from build123d import *

# Parameters (mm, degrees)
F0_R     = 15.875
F1_DEPTH = 12.7


with BuildPart() as f1:
    # F0 (on Top) → F1 (new body)
    with BuildSketch(Plane.XY):
        with BuildLine():
            ThreePointArc((139.501369, -7.447021), (139.650333, -3.724835), (139.7, 0))
            ThreePointArc((139.7, 0), (139.650333, 3.724835), (139.501369, 7.447021))
            ThreePointArc((139.501369, 7.447021), (132.862595, 43.169674), (117.236227, 75.97208))
            ThreePointArc((117.236227, 75.97208), (113.019674, 82.1136), (108.481729, 88.021614))
            ThreePointArc((108.481729, 88.021614), (82.1136, 113.019674), (50.190832, 130.37243))
            ThreePointArc((50.190832, 130.37243), (43.169674, 132.862595), (36.025756, 134.974942))
            ThreePointArc((36.025756, 134.974942), (0, 139.7), (-36.025756, 134.974942))
            ThreePointArc((-36.025756, 134.974942), (-43.169674, 132.862595), (-50.190832, 130.37243))
            ThreePointArc((-50.190832, 130.37243), (-82.1136, 113.019674), (-108.481729, 88.021614))
            ThreePointArc((-108.481729, 88.021614), (-113.019674, 82.1136), (-117.236227, 75.97208))
            ThreePointArc((-117.236227, 75.97208), (-132.862595, 43.169674), (-139.501369, 7.447021))
            ThreePointArc((-139.501369, 7.447021), (-139.7, 0), (-139.501369, -7.447021))
            ThreePointArc((-139.501369, -7.447021), (-132.862595, -43.169674), (-117.236227, -75.97208))
            ThreePointArc((-117.236227, -75.97208), (-113.019674, -82.1136), (-108.481729, -88.021614))
            ThreePointArc((-108.481729, -88.021614), (-82.1136, -113.019674), (-50.190832, -130.37243))
            ThreePointArc((-50.190832, -130.37243), (-43.169674, -132.862595), (-36.025756, -134.974942))
            ThreePointArc((-36.025756, -134.974942), (0, -139.7), (36.025756, -134.974942))
            ThreePointArc((36.025756, -134.974942), (43.169674, -132.862595), (50.190832, -130.37243))
            ThreePointArc((50.190832, -130.37243), (82.1136, -113.019674), (108.481729, -88.021614))
            ThreePointArc((108.481729, -88.021614), (113.019674, -82.1136), (117.236227, -75.97208))
            ThreePointArc((117.236227, -75.97208), (132.862595, -43.169674), (139.501369, -7.447021))
        make_face()
        Circle(F0_R, mode=Mode.SUBTRACT)
        with BuildLine():
            ThreePointArc((117.236227, 75.97208), (132.862595, 43.169674), (139.501369, 7.447021))
            Line((139.501369, 7.447021), (160.943947, 38.940288))
            Line((160.943947, 38.940288), (157.019431, 51.018706))
            Line((157.019431, 51.018706), (153.094915, 63.097124))
            Line((153.094915, 63.097124), (117.236227, 75.97208))
        make_face()
        with BuildLine():
            Line((160.943947, -38.940288), (139.501369, -7.447021))
            ThreePointArc((139.501369, -7.447021), (132.862595, -43.169674), (117.236227, -75.97208))
            Line((117.236227, -75.97208), (153.094915, -63.097124))
            Line((153.094915, -63.097124), (157.019431, -51.018706))
            Line((157.019431, -51.018706), (160.943947, -38.940288))
        make_face()
        with BuildLine():
            ThreePointArc((50.190832, 130.37243), (82.1136, 113.019674), (108.481729, 88.021614))
            Line((108.481729, 88.021614), (107.317861, 126.103833))
            Line((107.317861, 126.103833), (97.043345, 133.568706))
            Line((97.043345, 133.568706), (86.768829, 141.033578))
            Line((86.768829, 141.033578), (50.190832, 130.37243))
        make_face()
        with BuildLine():
            Line((107.317861, -126.103833), (108.481729, -88.021614))
            ThreePointArc((108.481729, -88.021614), (82.1136, -113.019674), (50.190832, -130.37243))
            Line((50.190832, -130.37243), (86.768829, -141.033578))
            Line((86.768829, -141.033578), (97.043345, -133.568706))
            Line((97.043345, -133.568706), (107.317861, -126.103833))
        make_face()
        with BuildLine():
            ThreePointArc((-36.025756, 134.974942), (0, 139.7), (36.025756, 134.974942))
            Line((36.025756, 134.974942), (12.7, 165.1))
            Line((12.7, 165.1), (0, 165.1))
            Line((0, 165.1), (-12.7, 165.1))
            Line((-12.7, 165.1), (-36.025756, 134.974942))
        make_face()
        with BuildLine():
            Line((12.7, -165.1), (36.025756, -134.974942))
            ThreePointArc((36.025756, -134.974942), (0, -139.7), (-36.025756, -134.974942))
            Line((-36.025756, -134.974942), (-12.7, -165.1))
            Line((-12.7, -165.1), (0, -165.1))
            Line((0, -165.1), (12.7, -165.1))
        make_face()
        with BuildLine():
            ThreePointArc((-108.481729, 88.021614), (-82.1136, 113.019674), (-50.190832, 130.37243))
            Line((-50.190832, 130.37243), (-86.768829, 141.033578))
            Line((-86.768829, 141.033578), (-97.043345, 133.568706))
            Line((-97.043345, 133.568706), (-107.317861, 126.103833))
            Line((-107.317861, 126.103833), (-108.481729, 88.021614))
        make_face()
        with BuildLine():
            Line((-86.768829, -141.033578), (-50.190832, -130.37243))
            ThreePointArc((-50.190832, -130.37243), (-82.1136, -113.019674), (-108.481729, -88.021614))
            Line((-108.481729, -88.021614), (-107.317861, -126.103833))
            Line((-107.317861, -126.103833), (-97.043345, -133.568706))
            Line((-97.043345, -133.568706), (-86.768829, -141.033578))
        make_face()
        with BuildLine():
            ThreePointArc((-139.501369, 7.447021), (-132.862595, 43.169674), (-117.236227, 75.97208))
            Line((-117.236227, 75.97208), (-153.094915, 63.097124))
            Line((-153.094915, 63.097124), (-157.019431, 51.018706))
            Line((-157.019431, 51.018706), (-160.943947, 38.940288))
            Line((-160.943947, 38.940288), (-139.501369, 7.447021))
        make_face()
        with BuildLine():
            Line((-153.094915, -63.097124), (-117.236227, -75.97208))
            ThreePointArc((-117.236227, -75.97208), (-132.862595, -43.169674), (-139.501369, -7.447021))
            Line((-139.501369, -7.447021), (-160.943947, -38.940288))
            Line((-160.943947, -38.940288), (-157.019431, -51.018706))
            Line((-157.019431, -51.018706), (-153.094915, -63.097124))
        make_face()
    extrude(amount=F1_DEPTH)


solid = f1.part
Can you work these out from the model? Positions are in its coordinate system, mm. A direction names the side the tool comes from. Give positions to 0.01 mm unless a question says otherwise; leave off trailing zeros. Loops run counter-clockwise (first coordinate to the right, second up) from the corner with the lowest first, then second, coordinate; pieces in that order, holes last. Notation, with made-up numbers: (60.25, 48) - (108.25, 48) arc R33 cw to (108.25, 77) - close; hole circle Ø1 at (16, 8). An arc over 180 degrees is marked (long way). Return JSON: item names as keys, results as strings.
1. We'd pull the mould along Y, two halves only. Please class faces 1 (the face through (-139.7, 0.1, 6.3)), 2 (the face through (-134.915, 69.625, 6.261)), 3 (the face through (156.964, -51.188, 6.261)): +Y half, -Y half, draft (parallel to the pull), parting line (faces both ways), or undercut.
Output values:
{"face 1": "undercut", "face 2": "+Y half", "face 3": "-Y half"}
2. For faces 4 (the face through (-43.27, -132.83, 6.26)), 5 (the face through (24.526, 149.827, 6.261)), 6 (the face through (-150.07, -22.97, 6.26)), 7 (the face through (150.07, 22.97, 6.26)), which set-ups out of +Z, -Z, +X, -X, +Y, -Y let a thin tool reach every point of the face, with its end or its side?
Output values:
{"face 4": "+Z, -Z, -Y", "face 5": "+Z, -Z, +Y", "face 6": "+Z, -Z, -X", "face 7": "+Z, -Z, +X"}
3. I'm going to push flat-ended pins straight in: pin 1 Ø6 at (x, z) = (20.5, 11.5) entering from +Y; pin 2 Ø3 at (y, z) = (-35, 7) entering from +X; pin 3 Ø4 at (y, z) = (-57, 10) entering from +X. Where does each tip first touch, or does it pass through?
Output values:
{"pin 1": "stops at y = 158.9", "pin 2": "stops at x = 159.28", "pin 3": "stops at x = 155.73"}
4. I want a section at A-A on x = 0. Please give me the cut outline in (y, z) (3 decimals), and give its area (3 significant figures).
Output values:
{"outline": "(-165.1, 0) - (-15.875, 0) - (-15.875, 12.7) - (-165.1, 12.7) - close; (15.875, 0) - (165.1, 0) - (165.1, 12.7) - (15.875, 12.7) - close", "area": "3,790 mm²"}
5. I want a section at B-B on y = 117.5. Please give me the cut outline in (x, z), and give its area (3 significant figures).
Output values:
{"outline": "(-107.58, 0) - (107.58, 0) - (107.58, 12.7) - (-107.58, 12.7) - close", "area": "2,730 mm²"}
6. I want a section at C-C on x = 78.5. Please give me the cut outline in (y, z), and give its area (3 significant figures).
Output values:
{"outline": "(-138.62, 0) - (138.62, 0) - (138.62, 12.7) - (-138.62, 12.7) - close", "area": "3,520 mm²"}
7. If I drill on line 1 (Y direction, x = 0, z = 9.75) (3 decimals); line 2 (Y direction, x = 95, z = 10.75); line 3 (X direction, y = 125, z = 2.25), over which ranges is the centre line in solid material (lowest first)?
Output values:
{"line 1": "y = -165.1 to -15.875, 15.875 to 165.1", "line 2": "y = -135.05 to 135.05", "line 3": "x = -107.35 to 107.35"}
